```python
from build123d import *

# Parameters (mm, degrees)
BOSS_EXTRU_1_DEPTH      = 3
ESQUISSE4_R             = 2
ENL_V_MAT_EXTRU_1_DEPTH = 10
BOSS_EXTRU_2_DEPTH      = 3
ESQUISSE6_W             = 163
ESQUISSE6_H             = 80
BOSS_EXTRU_3_DEPTH      = 3


with BuildPart() as part:
    # Esquisse2 → Boss.-Extru.1 (new body)
    with BuildSketch(Plane.XY):
        with BuildLine():
            Line((-57.997011135, -5.009122385), (105.002988865, -5.009122385))
            Line((105.002988865, -5.009122385), (105.002988865, -0.009122385))
            ThreePointArc((105.002988865, -0.009122385), (102.074056676, 7.061945427), (95.002988865, 9.990877615))
            Line((95.002988865, 9.990877615), (85.002988865, 9.990877615))
            Line((85.002988865, 9.990877615), (85.002988865, 9.996878601))
            ThreePointArc((85.002988865, 9.996878601), (82.076178664, 17.065823789), (75.008991651, 19.9968768))
            Line((75.008991651, 19.9968768), (-27.995184752, 20.058708021))
            Line((-27.995184752, 20.058708021), (-27.997011135, 20.058708021))
            ThreePointArc((-27.997011135, 20.058708021), (-35.068078947, 17.129775833), (-37.997011135, 10.058708021))
            Line((-37.997011135, 10.058708021), (-37.997011135, 9.990877615))
            Line((-37.997011135, 9.990877615), (-47.997011135, 9.990877615))
            ThreePointArc((-47.997011135, 9.990877615), (-55.068078947, 7.061945427), (-57.997011135, -0.009122385))
            Line((-57.997011135, -0.009122385), (-57.997011135, -5.009122385))
        make_face()
    extrude(amount=BOSS_EXTRU_1_DEPTH)

    # Esquisse4 → Enlèv. mat.-Extru.1 (cut)
    with BuildSketch(Plane.XY.offset(3)):
        with Locations((-32.497011135, 14.558708021)):
            Circle(ESQUISSE4_R)
        with Locations((79.502988865, 14.494178158)):
            Circle(ESQUISSE4_R)
        with Locations((99.502988865, 4.490877615)):
            Circle(ESQUISSE4_R)
        with Locations((-52.497011135, 4.490877615)):
            Circle(ESQUISSE4_R)
    extrude(amount=-ENL_V_MAT_EXTRU_1_DEPTH, mode=Mode.SUBTRACT)

    # Esquisse5 → Boss.-Extru.2 (add)
    with BuildSketch(Plane.XY.offset(3)):
        Polygon((-7.497011135, 20.046403402), (-7.497011135, 58.046403402), (54.502988865, 58.046403402), (54.502988865, 20.009186118), align=None)
    extrude(amount=-BOSS_EXTRU_2_DEPTH)

    # Esquisse6 → Boss.-Extru.3 (add)
    with BuildSketch(Plane.XY.offset(3)):
        with Locations((23.502988865, -45.009122385)):
            Rectangle(ESQUISSE6_W, ESQUISSE6_H)
    extrude(amount=-BOSS_EXTRU_3_DEPTH)


solid = part.part
```
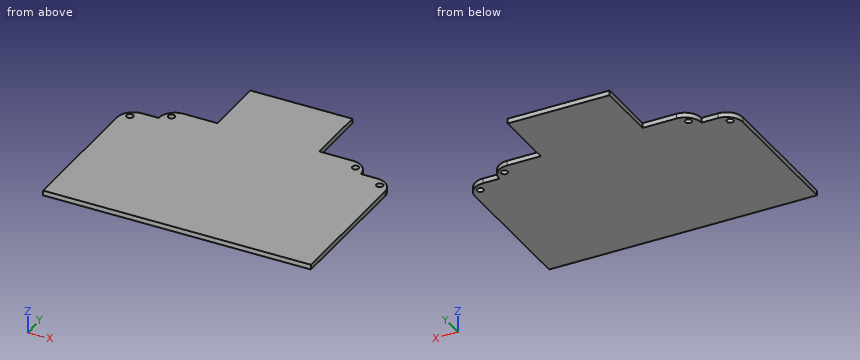
Geometry check sheet. Reference: the model listing, model coordinates, mm. Coordinates: 2 decimals unless noted, no trailing zeros. Order: outer loops, then holes, each group sorted by start corner. A loop starts at its lowest first (then second) coordinate and runs counter-clockwise, first axis right, second up. Notation, with made-up numbers: M -27.5,50 L 18.5,50 A19 ccw 18.5,63 Z; hole C 21.25,26 d5. An arc over 180 degrees is marked long. One line per question, with ' | ' between items. Start each with the question number.
Item 1: Cross-section at B-B on z = 1.6. State how many separate pieces and enclosed holes the cut face has, then the cut area to 3 significant figures.
Item 2: Material ranges on L1, parallel to X at y = 15, z = 1.25; L2, parallel to X at y = 39, z = 2.7; L3, parallel to Y at x = -10.5, z = 0.35, recorded low to high. Write a range as [from, to].
Item 3: Gauge pin test, flat ends, axial feed: pin 1 (4.5 mm diameter, centred on x = -52.5, y = 4.49, fed in from -Z); pin 2 (3 mm diameter, centred on x = -32.5, y = 14.56, fed in from -Z); pin 3 (0.9 mm diameter, centred on x = 88, z = 1, fed in from +Y); pin 4 (0.9 mm diameter, centred on y = 33.5, z = 1.5, fed in from +X). Record the tip position at first contact, or that the pin passes through.
Item 4: Cross-section at A-A on x = 89. Enter the section's corners in (y, z).
Findings:
1) separate pieces: 1 | enclosed holes: 4 | area: 18,900 mm²
2) L1: x = [-36.69, -34.45], [-30.55, 77.57], [81.44, 83.66] | L2: x = [-7.5, 54.5] | L3: y = [-85.01, 20.05]
3) pin 1: stops at z = 0 | pin 2: passes through | pin 3: stops at y = 9.99 | pin 4: stops at x = 54.5
4) outline: M -85.01,0 L 9.99,0 L 9.99,3 L -85.01,3 Z
